```python
from build123d import *

# Parameters (mm, degrees)
SKETCH1_W           = 13
SKETCH1_H           = 7.5
SKETCH1_W_2         = 11
SKETCH1_H_2         = 5.5
BOSS_EXTRUDE1_DEPTH = 7.75
SKETCH2_R           = 2.75
CUT_EXTRUDE1_DEPTH  = 1
SKETCH3_W           = 13
SKETCH3_H           = 7.5
BOSS_EXTRUDE2_DEPTH = 1
BOSS_EXTRUDE3_DEPTH = 3


with BuildPart() as part:
    # Sketch1 → Boss-Extrude1 (new body)
    with BuildSketch(Plane(origin=(0, 0, 0), x_dir=(1, 0, 0), z_dir=(0, 1, 0))):
        Rectangle(SKETCH1_W, SKETCH1_H)
        Rectangle(SKETCH1_W_2, SKETCH1_H_2, mode=Mode.SUBTRACT)
    extrude(amount=BOSS_EXTRUDE1_DEPTH)

    # Sketch2 → Cut-Extrude1 (cut)
    with BuildSketch(Plane.ZY.offset(6.5)):
        with Locations((0, 3.75)):
            Circle(SKETCH2_R)
    extrude(amount=-CUT_EXTRUDE1_DEPTH, mode=Mode.SUBTRACT)

    # Sketch3 → Boss-Extrude2 (add)
    with BuildSketch(Plane.XZ):
        Rectangle(SKETCH3_W, SKETCH3_H)
    extrude(amount=-BOSS_EXTRUDE2_DEPTH)

    # Sketch4 → Boss-Extrude3 (add, symmetric)
    with BuildSketch(Plane.XY):
        Polygon((2.25, 1), (5.5, 6.5), (5.5, 1), align=None)
    extrude(amount=BOSS_EXTRUDE3_DEPTH, both=True)


solid = part.part
```
Here's how the part is built. I have some questions about the finished solid (model axes, mm). A direction names the side the tool comes from. Coordinates: 2 decimals unless noted, no trailing zeros. Order: outer loops, then holes, each group sorted by start corner. A loop starts at its lowest first (then second) coordinate and runs counter-clockwise, first axis right, second up. Notation, with made-up numbers: (-6.75, 61.25) - (46.25, 61.25) arc R10 ccw to (46.25, 74.25) - close; hole circle Ø9 at (-8.75, -0.5). An arc over 180 degrees is marked (long way). One line per question, with ' | ' between items. Start each with the question number.
1. Please list where these lines run through material, in increasing order: line 1 along Y through (x, z) = (-6.05, 0); line 2 along Z through (x, y) = (-6.3, 3.75). Write a range as [from, to].
2. I'm going to push a flat-ended pin straight in: pin 1 Ø1.6 at (x, z) = (-1.5, 0.5) entering from +Y. Where does the tip first touch, or does it pass through?
3. If we section it at A-A (z = 2): Write out the boundary of the cut face in (x, y), and give its area (3 significant figures).
4. Which directions (+Z, -Z, +X, -X, +Y, -Y) give clear straight access to the entire face, cutting with the end or side of a thin tool? Please do faces 1 (the flat face through (0, 7.75, 3)), 2 (the flat face through (-5.5, 7, 0)), 3 (the cylindrical face through (-6.007, 1.065, -0.596)).
5. If we section it at B-B (x = -1.5): Write out the boundary of the cut face in (y, z).
6. If we mould it in two halves opening along X, with no side actions, what happens to faces 4 (the flat face through (6.5, 4, 0)), 5 (the flat face through (0, 4, 2.75)), 6 (the flat face through (0, 0, 0)), 7 (the flat face through (5.5, 7, 0))? For each: released by +X, released by -X, zero draft, split by the parting line, or undercut.
7. If we section it at D-D (z = 0.75): Write out the boundary of the cut face in (x, y), and give its area (3 significant figures).
8. If we section it at C-C (y = 2.75): Write out the boundary of the cut face in (x, z), and give its area (3 significant figures).
Model answer:
1) line 1: y = [0, 1], [6.5, 7.75] | line 2: z = [-3.75, -2.75], [2.75, 3.75]
2) pin 1: stops at y = 1
3) outline: (-6.5, 0) - (6.5, 0) - (6.5, 7.75) - (5.5, 7.75) - (5.5, 6.5) - (2.25, 1) - (-5.5, 1) - (-5.5, 1.86) - (-6.5, 1.86) - close; (-6.5, 5.64) - (-5.5, 5.64) - (-5.5, 7.75) - (-6.5, 7.75) - close | area: 31.7 mm²
4) face 1: +Z, -Z, +X, -X, +Y | face 2: +Y | face 3: -X
5) outline: (0, -3.75) - (7.75, -3.75) - (7.75, -2.75) - (1, -2.75) - (1, 2.75) - (7.75, 2.75) - (7.75, 3.75) - (0, 3.75) - close
6) face 4: released by +X | face 5: undercut | face 6: zero draft | face 7: undercut
7) outline: (-6.5, 0) - (6.5, 0) - (6.5, 7.75) - (5.5, 7.75) - (5.5, 6.5) - (2.25, 1) - (-5.5, 1) - (-5.5, 1.1) - (-6.5, 1.1) - close; (-6.5, 6.4) - (-5.5, 6.4) - (-5.5, 7.75) - (-6.5, 7.75) - close | area: 30.1 mm²
8) outline: (-6.5, -3.75) - (6.5, -3.75) - (6.5, 3.75) - (-6.5, 3.75) - (-6.5, 2.56) - (-5.5, 2.56) - (-5.5, 2.75) - (3.28, 2.75) - (3.28, -2.75) - (-5.5, -2.75) - (-5.5, -2.56) - (-6.5, -2.56) - close | area: 44.1 mm²
